Could you check a few things on this drawing? It's one solid part, dimensions in mm from its lowest x, y, z. A direction names the side the tool comes from. Give positions to 0.01 mm unless a question says otherwise; leave off trailing zeros. Loops run counter-clockwise (first coordinate to the right, second up) from the corner with the lowest first, then second, coordinate; pieces in that order, holes last. Notation, with made-up numbers: (-7.75, 23) - (6.25, 23) arc R20 ccw to (6.25, 53) - close; hole circle Ø2 at (-7, -15). An arc over 180 degrees is marked (long way). Return JSON: item names as keys, results as strings. Group by question number.
(1) I need wall thicknesses on probe 1 along X at (y, z) = (3.7, 5); probe 2 along X at (y, z) = (0.45, 18.25); probe 3 along Z at (x, y) = (7.5, 2.5). Which ranges of each line are inside material? Lowest first, please. Write a range as [from, to].
(2) For P1, Ø3, axis at x = 29, z = 5, coming from the -Y side, with a flat end and sliding along its axis, tell me the tip position at first contact or that it passes through.
(3) If we mould it in two halves opening along Z, with no side actions, what happens to the marked faces 1, 2 and 3? For each: released by +Z, released by -Z, zero draft, split by the parting line, or undercut.
(4) If we section it at C-C (y = 3.95): Please give me the cut outline in (x, z).
(5) If we section it at B-B (x = 21): Please give me the cut outline in (y, z), then the cut area to 3 significant figures.
(6) If we section it at D-D (z = 5): Please give me the cut outline in (x, y), then the cut area to 3 significant figures.
(7) If we section it at A-A (z = 14): Please give me the cut outline in (x, y), then the cut area to 3 significant figures.
(8) On a 3-axis mill with a long thin cutter (end or side, diameter ignored), from which of +Z, -Z, +X, -X, +Y, -Y can I reach the whole of each face in a straight line? I mean the marked faces 4 and 5. Say none if no direction works.
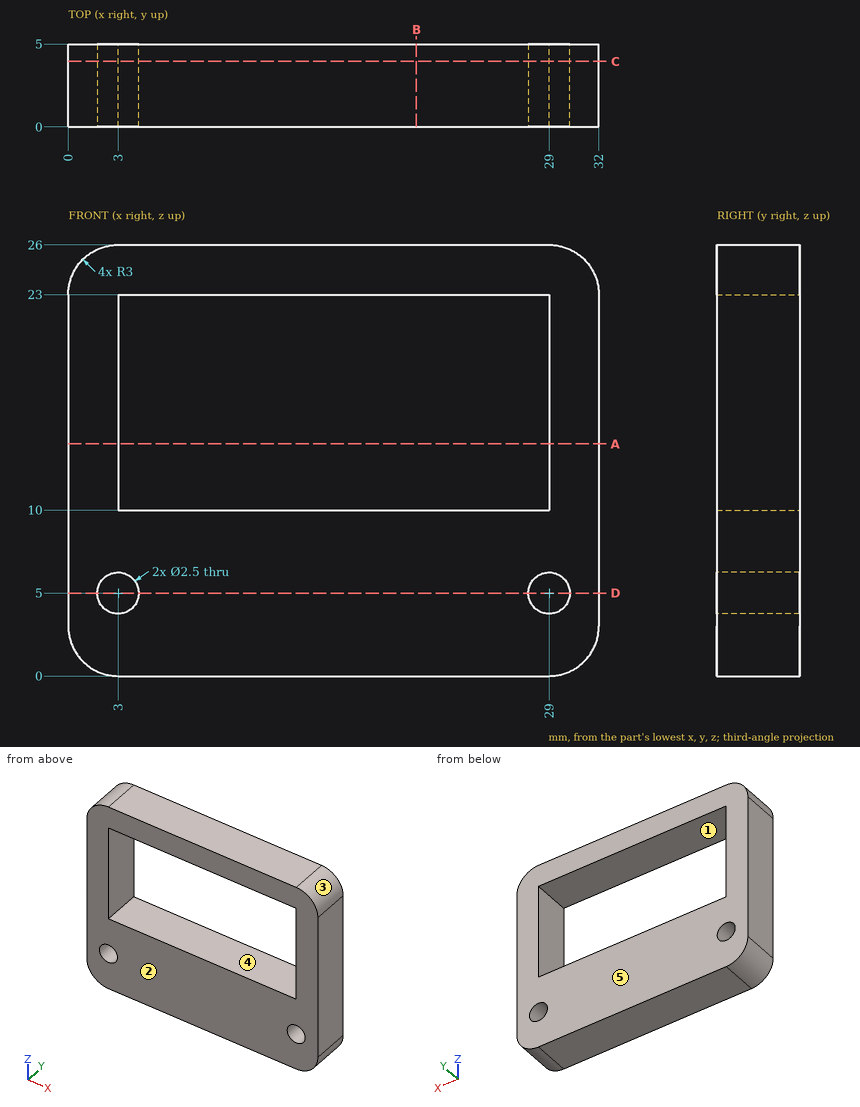
Values:
{
 "1": {"probe 1": "[0, 1.75], [4.25, 27.75], [30.25, 32]", "probe 2": "[0, 3], [29, 32]", "probe 3": "[0, 10], [23, 26]"},
 "2": {"P1": "y = 0"},
 "3": {"face 1": "undercut", "face 2": "zero draft", "face 3": "released by +Z"},
 "4": {"outline": "(0, 3) arc R3 ccw to (3, 0) - (29, 0) arc R3 ccw to (32, 3) - (32, 23) arc R3 ccw to (29, 26) - (3, 26) arc R3 ccw to (0, 23) - close; hole circle Ø2.5 at (3, 5); hole (3, 10) - (29, 10) - (29, 23) - (3, 23) - close; hole circle Ø2.5 at (29, 5)"},
 "5": {"outline": "(0, 0) - (5, 0) - (5, 10) - (0, 10) - close; (0, 23) - (5, 23) - (5, 26) - (0, 26) - close", "area": "65.0 mm2"},
 "6": {"outline": "(0, 0) - (1.75, 0) - (1.75, 5) - (0, 5) - close; (4.25, 0) - (27.75, 0) - (27.75, 5) - (4.25, 5) - close; (30.25, 0) - (32, 0) - (32, 5) - (30.25, 5) - close", "area": "135 mm2"},
 "7": {"outline": "(0, 0) - (3, 0) - (3, 5) - (0, 5) - close; (29, 0) - (32, 0) - (32, 5) - (29, 5) - close", "area": "30.0 mm2"},
 "8": {"face 4": "+Y, -Y", "face 5": "+Z, -Z, +X, -X, +Y"}
}
